The listing builds one solid part. Answer for the finished solid, in the listing's coordinates (mm). Give positions to 0.01 mm unless a question says otherwise; leave off trailing zeros. Write each loop counter-clockwise with the first axis right and the second up, starting at its lowest first coordinate (ties: lowest second). Pieces come first, ordered by that corner, then holes. Notation, with made-up numbers: M 16,19.5 L 24,19.5 A17 ccw 24,27.5 Z; hole C 87,4.5 d11. An arc over 180 degrees is marked long. Return JSON: item names as keys, results as strings.
Autodesk Inventor part; units mm, degrees
ref_plane "YZ Plane" through (0, 0, 0) normal (1, 0, 0) x (0, 1, 0)
ref_plane "XZ Plane" through (0, 0, 0) normal (0, 1, 0) x (-1, 0, 0)
ref_plane "XY Plane" through (0, 0, 0) normal (0, 0, 1) x (1, 0, 0)
sketch "Sketch1" plane through (0, 0, 0) normal (0, 1, 0) x (-1, 0, 0)
  line L0 (0, 0) -> (50, 0)
  line L1 (50, 0) -> (50, -58)
  line L2 (50, -58) -> (0, -58)
  line L3 (0, -58) -> (0, 0)
  circle A0 centre (41.4991, -7.5) radius 2.5
  circle A1 centre (41.4991, -51) radius 2.5
  circle A2 centre (8.5, -50.75) radius 2.5
  circle A3 centre (8.5, -7.25) radius 2.5
  dimension "d0" = 50
  dimension "d1" = 58
  dimension "d2" = 5
  dimension "d3" = 5
  dimension "d4" = 5
  dimension "d5" = 5
  dimension "d7" = 8.5
  dimension "d8" = 33
  dimension "d9" = 33
  dimension "d10" = 7.25
  dimension "d11" = 7
  dimension "d14" = 43.5
  dimension "d15" = 43.5
extrude "Extrusion1" add sketch "Sketch1" along normal blind 2
fillet "Fillet1" radius 3 4 edges at (-50, 1, -58) (0, 1, -58) (0, 1, 0) (-50, 1, 0)
properties part number "PCB_design"
Item 1: Determine the mould class of faces 1 (the cylindrical face through (-9.65, 0.99, -5.03)), 2 (the cylindrical face through (-49.14, 1.01, -0.9)), 3 (the flat face through (0, 1, -29)) for opening direction X: +X half, -X half, draft (parallel to the pull), parting line (faces both ways), or undercut.
Geometry results:
{"face 1": "undercut", "face 2": "-X half", "face 3": "+X half"}
Item 2: A cutting plane is placed at A-A, the plane x = -8.5. Write down the section's boundary in (y, z).
Geometry results:
{"outline": "M 0,-58 L 2,-58 L 2,-53.25 L 0,-53.25 Z; M 0,-48.25 L 2,-48.25 L 2,-9.75 L 0,-9.75 Z; M 0,-4.75 L 2,-4.75 L 2,0 L 0,0 Z"}
Item 3: A cutting plane is placed at C-C, the plane z = -52. Write down the section's boundary in (x, y).
Geometry results:
{"outline": "M -50,0 L -43.79,0 L -43.79,2 L -50,2 Z; M -39.21,0 L -10.67,0 L -10.67,2 L -39.21,2 Z; M -6.33,0 L 0,0 L 0,2 L -6.33,2 Z"}
Item 4: Given pin 1 Ø3 at (x, z) = (-8.5, -7.25) entering from +Y, flat-ended and moving along its own axis, determine where the tip first touches the part or whether it passes through.
Geometry results:
{"pin 1": "passes through"}
Item 5: Find the intervals of material crossed by line 1 (Z direction, x = -8.5, y = 1.3); line 2 (Z direction, x = -43.5, y = 1.05), in increasing order.
Geometry results:
{"line 1": "z = -58 to -53.25, -48.25 to -9.75, -4.75 to 0", "line 2": "z = -58 to -52.5, -49.5 to -9, -6 to 0"}
Item 6: A cutting plane is placed at B-B, the plane y = 1.65. Write down the section's boundary in (x, z), plus the area to 3 significant figures.
Geometry results:
{"outline": "M -50,-55 A3 ccw -47,-58 L -3,-58 A3 ccw 0,-55 L 0,-3 A3 ccw -3,0 L -47,0 A3 ccw -50,-3 Z; hole C -41.5,-51 d5; hole C -41.5,-7.5 d5; hole C -8.5,-50.75 d5; hole C -8.5,-7.25 d5", "area": "2,810 mm2"}
